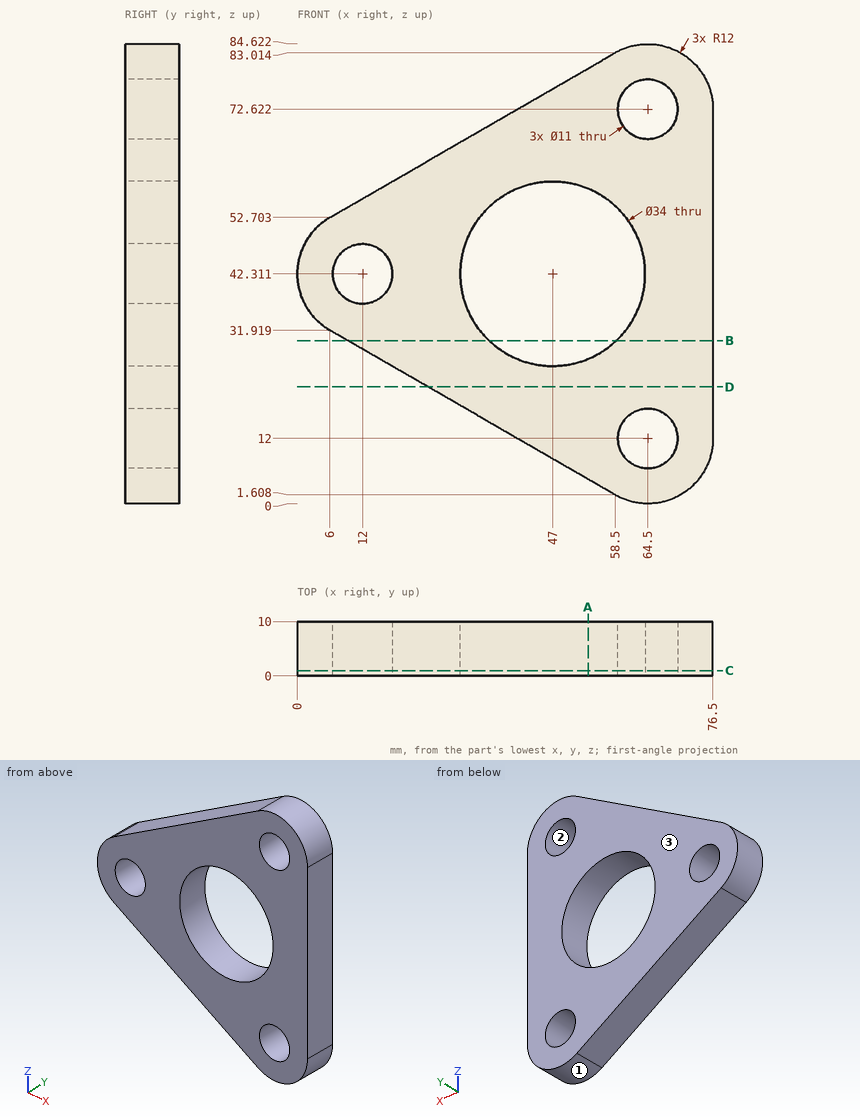
Could you check a few things on this drawing? It's one solid part, dimensions in mm from its lowest x, y, z. Coordinates: 2 decimals unless noted, no trailing zeros. Loops run counter-clockwise (first coordinate to the right, second up) from the corner with the lowest first, then second, coordinate; pieces in that order, holes last.
1. We'd pull the mould along Z, two halves only. Please class the marked faces 1, 2 and 3: released by +Z, released by -Z, zero draft, split by the parting line, or undercut.
2. Imagine slicing it at D-D (z = 21.5). Please give me the cut outline in (x, y) (1 decimal).
3. Imagine slicing it at A-A (x = 53.5). Please give me the cut outline in (y, z) (1 decimal).
4. For P1, Ø20.5, axis at x = 47, z = 42.31, coming from the -Y side; P2, Ø2, axis at y = 8, z = 24.5, coming from the -X side (1 decimal); P3, Ø2, axis at y = 9, z = 29.5, coming from the -X side (1 decimal), each with a flat end and sliding along its axis, tell me the tip position at first contact or that it passes through.
5. Imagine slicing it at B-B (z = 30). Please give me the cut outline in (x, y), and give its area (3 significant figures).
6. I need wall thicknesses on L1, parallel to Z at x = 64.5, y = 5.5; L2, parallel to Z at x = 65.5, y = 2; L3, parallel to X at y = 7, z = 48 (1 decimal). Which ranges of each line are inside material? Lowest first, please.
7. Imagine slicing it at C-C (y = 1). Please give me the cut outline in (x, z) (1 decimal).
Computed values:
1. face 1: released by -Z
1. face 2: undercut
1. face 3: zero draft
2. outline: (24, 0) - (76.5, 0) - (76.5, 10) - (24, 10) - close
3. outline: (0, 4.5) - (10, 4.5) - (10, 26.6) - (0, 26.6) - close; (0, 58) - (10, 58) - (10, 80.1) - (0, 80.1) - close
4. P1: passes through
4. P2: stops at x = 17.1
4. P3: stops at x = 8.5
5. outline: (9.32, 0) - (35.28, 0) - (35.28, 10) - (9.32, 10) - close; (58.72, 0) - (76.5, 0) - (76.5, 10) - (58.72, 10) - close
5. area: 437 mm2
6. L1: z = 0 to 6.5, 17.5 to 67.12, 78.12 to 84.62
6. L2: z = 0.04 to 6.59, 17.41 to 67.21, 78.03 to 84.58
6. L3: x = 1.4 to 31, 63 to 76.5
7. outline: (6, 31.9) - (58.5, 1.6) arc R12 ccw to (76.5, 12) - (76.5, 72.6) arc R12 ccw to (58.5, 83) - (6, 52.7) arc R12 ccw to start; hole circle Ø11 at (12, 42.3); hole circle Ø34 at (47, 42.3); hole circle Ø11 at (64.5, 12); hole circle Ø11 at (64.5, 72.6)
